```python
from build123d import *

# Parameters (mm, degrees)
F0_W     = 112.000551
F0_H     = 85.980557
F1_DEPTH = 100
F3_D     = 12
F4_R     = 12.259928
F5_DEPTH = 4


with BuildPart() as f1:
    # F0 (on Top) → F1 (new body)
    with BuildSketch(Plane.XY):
        with Locations((11.973376, -18.311291)):
            Rectangle(F0_W, F0_H)
    extrude(amount=F1_DEPTH)

    # F3 (through all)
    with Locations(Plane.XY.offset(100)):
        with Locations((9.428112, -18.311292)):
            Hole(F3_D / 2)

    # F4 (on face) → F5 (cut)
    with BuildSketch(Plane.XY.offset(100)):
        with Locations((9.428112, -18.311292)):
            Circle(F4_R)
    extrude(amount=-F5_DEPTH, mode=Mode.SUBTRACT)


solid = f1.part
```
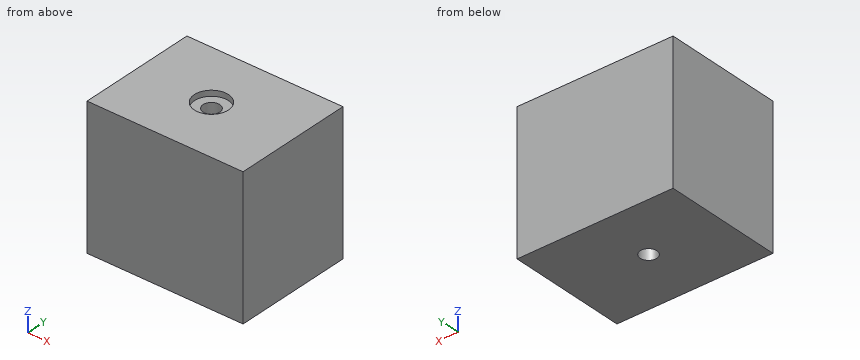
Model file for the job. Use its own axes, mm. Give positions to 0.01 mm unless a question says otherwise; leave off trailing zeros. Loops run counter-clockwise (first coordinate to the right, second up) from the corner with the lowest first, then second, coordinate; pieces in that order, holes last. Notation, with made-up numbers: M 56.25,-12 L 60.25,-12 A13 ccw 60.25,1 Z; hole C 5.5,21.25 d11. An arc over 180 degrees is marked long. Use one line per item in the form item = value.
Item 1: Slice it at A-A on y = -15. List the corners of the cut face in (x, z).
Filled in:
outline = M -44.03,0 L 4.42,0 L 4.42,96 L -2.38,96 L -2.38,100 L -44.03,100 Z; M 14.43,0 L 67.97,0 L 67.97,100 L 21.23,100 L 21.23,96 L 14.43,96 Z
Item 2: Drill centre lines: L1, parallel to Y at x = 9, z = 44; L2, parallel to X at y = -13, z = 17. Where is each one in solid material? Low to high.
Filled in:
L1 = -61.3 to -24.3, -12.33 to 24.68
L2 = -44.03 to 6.64, 12.22 to 67.97
Item 3: Flat gauge pins, fed straight in: pin 1 Ø10 at (x, y) = (43, 15.5) entering from -Z; pin 2 Ø19 at (x, y) = (9.43, -18.31) entering from +Z. Where does each tip first touch, or does it go through?
Filled in:
pin_1 = 0
pin_2 = 96
